Work out the finished part from the listing and answer in its coordinate system (mm). Face numbers are marked on the shaded views. Give positions to 0.01 mm unless a question says otherwise; leave off trailing zeros. Order: outer loops, then holes, each group sorted by start corner. A loop starts at its lowest first (then second) coordinate and runs counter-clockwise, first axis right, second up. Notation, with made-up numbers: (8, -23.75) -> (18, -23.75) arc R18 ccw to (18, 6.25) -> close; hole circle Ø2 at (-24.5, -39). An arc over 180 degrees is marked (long way). Answer as CSV lines item,"result". Start each with the question number.
1. A cutting plane is placed at C-C (z = -1.5). Give the vertices of the cut face in (x, y), then the cut area to 3 significant figures.
2. Find the intervals of material crossed by L1, parallel to Y at x = 0, z = 1.3; L2, parallel to Y at x = 1.15, z = 0.8; L3, parallel to X at y = 0.2, z = -0.95, in increasing order.
3. For a pull along X with two mould halves and no side action, classify the marked faces 1, 2 and 3 as released by +X, released by -X, zero draft, split by the parting line, or undercut.
4. A cutting plane is placed at A-A (y = 0). Give the vertices of the cut face in (x, z).
Solid Edge part; units mm, degrees
sketch "Sketch1" plane through (0, 0, 0) normal (0, 0, 1) x (1, 0, 0)
  circle A0 centre (0, 0) radius 2.5
  circle A1 centre (0, 0) radius 1.6
extrude "ExtrudedProtrusion_1" add sketch "Sketch1" along normal mid plane 6
fillet "Round_1" radius 0.2 4 edges at (-1.6, 0, 3) (-2.5, 0, 3) (-1.6, 0, -3) (-2.5, 0, -3)
properties material "Acrylic, high impact grade"
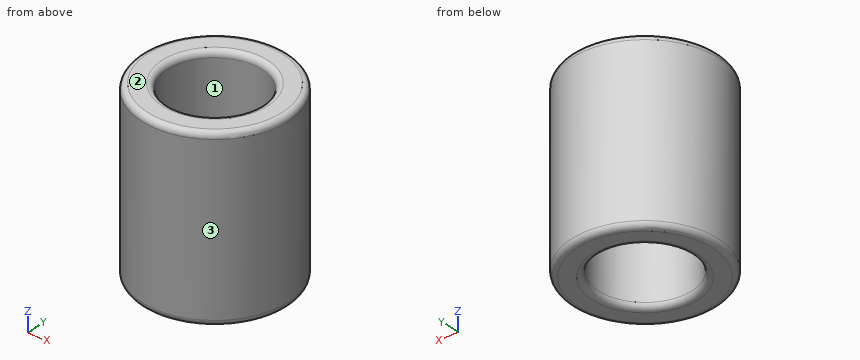
Answer sheet:
1,outline,"circle Ø5 at (0, 0); hole circle Ø3.2 at (0, 0)"
1,area,"11.6 mm^2"
2,L1,"y = -2.5 to -1.6, 1.6 to 2.5"
2,L2,"y = -2.22 to -1.11, 1.11 to 2.22"
2,L3,"x = -2.49 to -1.59, 1.59 to 2.49"
3,face 1,"undercut"
3,face 2,"zero draft"
3,face 3,"split by the parting line"
4,outline,"(-2.5, -2.8) arc R0.2 ccw to (-2.3, -3) -> (-1.8, -3) arc R0.2 ccw to (-1.6, -2.8) -> (-1.6, 2.8) arc R0.2 ccw to (-1.8, 3) -> (-2.3, 3) arc R0.2 ccw to (-2.5, 2.8) -> close; (1.6, -2.8) arc R0.2 ccw to (1.8, -3) -> (2.3, -3) arc R0.2 ccw to (2.5, -2.8) -> (2.5, 2.8) arc R0.2 ccw to (2.3, 3) -> (1.8, 3) arc R0.2 ccw to (1.6, 2.8) -> close"
